Work out the finished part from the listing and answer in its coordinate system (mm). A direction names the side the tool comes from. Round coordinates to 2 decimals unless told otherwise and drop trailing zeros. Write each loop counter-clockwise with the first axis right and the second up, starting at its lowest first coordinate (ties: lowest second). Pieces come first, ordered by that corner, then holes. Notation, with made-up numbers: (24, 7.25) - (56, 7.25) arc R6 cw to (56, 14.25) - close; hole circle Ø11 at (-39.75, 17). An arc over 180 degrees is marked (long way). Write item = value, one per line. Start each with the question number.
Autodesk Inventor part; units mm, degrees
ref_plane "Arbeitsebene1" through (50, 151.9868, 0) normal (-1, 0, 0) x (0, 0, 1)
ref_plane "YZ Plane" through (0, 0, 0) normal (1, 0, 0) x (0, 1, 0)
ref_plane "XZ Plane" through (0, 0, 0) normal (0, 1, 0) x (-1, 0, 0)
sketch "Skizze1" plane through (0, 0, 0) normal (0, 0, 1) x (1, 0, 0)
  line L0 (-33.0017, 0) -> (83.0017, 0) construction
  circle A0 centre (50, 151.9868) radius 16
  line L1 (66, 151.9868) -> (66, 221.9868)
  line L2 (34, 151.9868) -> (34, 221.9868)
  line L3 (50, 151.9868) -> (50, 237.9868) construction
  line L4 (50, 151.9868) -> (50, 167.9868) construction
  line L5 (34, 151.9868) -> (66, 151.9868) construction
  line L6 (-16, 0) -> (-16, 50)
  line L7 (16, 0) -> (16, 50)
  line L8 (-16, 50) -> (16, 50) construction
  circle A1 centre (0, 50) radius 16 construction
  line L9 (-14.2566, 57.2629) -> (34, 151.9868)
  arc A2 (-14.2566, 57.2629) -> (-16, 50) centre (0, 50) ccw
  line L10 (16, 50) -> (64.2566, 144.7239)
  arc A3 (64.2566, 144.7239) -> (66, 151.9868) centre (50, 151.9868) ccw
  line L11 (0, 50) -> (50, 151.9868) construction
  circle A4 centre (50, 221.9868) radius 16
  circle A5 centre (50, 221.9868) radius 9.5
  circle A6 centre (50, 151.9868) radius 9.5
  line L12 (0, 0) -> (0, 5) construction
  circle A7 centre (50, 151.9868) radius 12.75 construction
  circle A8 centre (50, 221.9868) radius 12.75 construction
  line L13 (0, 0) -> (50, 221.9868) construction
  circle A9 centre (50, 221.9868) radius 10.5
  circle A10 centre (50, 151.9868) radius 10.5
  circle A11 centre (50, 151.9868) radius 12
  circle A12 centre (50, 221.9868) radius 12
  line L14 (-16, 0) -> (-16, -17)
  line L15 (-16, -17) -> (16, -17)
  line L16 (16, -17) -> (16, 0)
  circle A13 centre (0, 0) radius 5
  line L17 (-1.5, -4.7697) -> (-1.5, -17)
  line L18 (1.5, -17) -> (1.5, -4.7697)
  line L19 (-16, 0) -> (16, 0) construction
  arc A14 (16, 0) -> (-16, 0) centre (0, 0) ccw
  line L20 (-1.5, 4.7697) -> (-1.5, 10.7697)
  arc A15 (1.5, 10.7697) -> (-1.5, 10.7697) centre (0, 10.7697) ccw
  line L21 (1.5, 10.7697) -> (1.5, 4.7697)
  line L22 (1.5, 4.7697) -> (-1.5, 4.7697)
  line L23 (0, 12.2697) -> (0, 40)
  line L24 (0, 40) -> (16, 40)
  line L25 (0, 33) -> (-4.8, 35)
  line L26 (-4.8, 35) -> (-4.8, 21)
  line L27 (-4.8, 21) -> (0, 23)
  line L28 (-4.8, 28) -> (0, 28) construction
  line L29 (-4.8, 30.5) -> (0, 30.5) construction
  line L30 (-4.8, 25.5) -> (0, 25.5) construction
  circle A16 centre (-10.5, 0) radius 1.55
  circle A17 centre (10.5, 0) radius 1.55
  line L31 (0, 0) -> (50, 151.9868) construction
  point P0 (26.4122, 103.8739)
  point P1 (50, 186.9868)
  point P2 (50, 164.7368)
  point P3 (38.9582, 145.6118)
  point P4 (61.0418, 145.6118)
  point P5 (50, 234.7368)
  point P6 (38.9582, 215.6118)
  point P7 (61.0418, 215.6118)
  point P8 (-5, 0)
  dimension "d69" = 25.5
  dimension "ParallelHebel_Passflansch_HoleDia" = 25.5
  dimension "d36" = 0
  dimension "ParallelHebel_Gabelgelenk_OuterDia" = 32
  dimension "VerticalDistance" = 70
  dimension "d42" = 60
  dimension "d43" = 19
  dimension "Nadellager_OuterDia" = 19
  dimension "d45" = 35
  dimension "d67" = 360
  dimension "d72" = 360
  dimension "Distanze_daVinciHead_Pivot" = 221.9868
  dimension "d88" = 21
  dimension "d91" = 24
  dimension "d92" = 24
  dimension "d97" = 151.9868
  dimension "Support_Link_Length" = 160
  dimension "d100" = 10
  dimension "d101" = 3
  dimension "d102" = 0
  dimension "d103" = 17
  dimension "d105" = 32
  dimension "d125" = 50
  dimension "d128" = 50
  dimension "d138" = 6
  dimension "d139" = 10
  dimension "d142" = 14
  dimension "d143" = 10
  dimension "d144" = 2.5
  dimension "d145" = 5
  dimension "d146" = 4.8
  dimension "d147" = 28
  dimension "d173" = 11
  dimension "d174" = 5.5
  dimension "d175" = 3.1
  dimension "d178" = 71.79
extrude "Extrusion2" add sketch "Skizze1" along normal blind 8 contours A0 | A0 L2 A4 L1 | A0 L10 L7 L24 L23 L25 L26 L27 A14 L6 A2 L9 | A4 | L7 A14 L23 L24 | A14 L23 A15 L20 A13 L17 L15 L14 | L16 L15 L18 A13 L21 A15 L23 A14 | L23 L27 L26 L25 | A15 L21 A13 L20 | A9 | A10 | A11 | A12 | A16 | A17
fillet "Rundung1" radius 25 2 edges at (34, 151.9868, 4) (16, 50, 4)
hole "Bohrung2" at (50, 186.9868, 0) at (26.4122, 103.8739, 0) direction (0, 0, 1) diameter 8 end through all
ref_plane "Arbeitsebene1" through (50, 151.9868, 0) normal (-1, 0, 0) x (0, 0, 1)
extrude "Extrusion6" cut sketch "Skizze1" along normal blind 1 contours A5 | A9 | A10 | A11 | A12
extrude "Extrusion7" cut sketch "Skizze1" along normal blind 1 from surface at 1 contours A9 | A10
sketch "Skizze8" plane through (0, 0, 8) normal (0, 0, 1) x (1, 0, 0)
  circle A0 centre (50, 186.9868) radius 4
  circle A1 centre (26.4122, 103.8739) radius 4
  arc A2 (64.2566, 144.7239) -> (66, 151.9868) centre (50, 151.9868) ccw
  line L0 (66, 151.9868) -> (66, 221.9868)
  arc A3 (66, 221.9868) -> (34, 221.9868) centre (50, 221.9868) ccw
  line L1 (34, 221.9868) -> (34, 157.988)
  arc A4 (31.2759, 146.6396) -> (34, 157.988) centre (9, 157.988) ccw
  line L2 (31.2759, 146.6396) -> (-14.2566, 57.2629)
  arc A5 (-14.2566, 57.2629) -> (-16, 50) centre (0, 50) ccw
  line L3 (-16, 50) -> (-16, -17)
  line L4 (-16, -17) -> (-1.5, -17)
  line L5 (-1.5, -17) -> (-1.5, -4.7697)
  arc A6 (1.5, -4.7697) -> (-1.5, -4.7697) centre (0, 0) ccw
  line L6 (1.5, -4.7697) -> (1.5, -17)
  line L7 (1.5, -17) -> (16, -17)
  line L8 (16, -17) -> (16, 43.9989)
  arc A7 (18.7241, 55.3472) -> (16, 43.9989) centre (41, 43.9989) ccw
  line L9 (18.7241, 55.3472) -> (64.2566, 144.7239)
  circle A8 centre (50, 151.9868) radius 9.5
  circle A9 centre (50, 221.9868) radius 9.5
extrude "Extrusion9" add sketch "Skizze8" along normal blind 5
sketch "Skizze5" plane through (-1.5, -17, 0) normal (1, 0, 0) x (0, 0, -1)
  line L0 (0, 0) -> (0, 12.2303) construction
  line L1 (0, 12.2303) -> (-13, 12.2303) construction
  line L2 (0, 0) -> (-13, 0) construction
  line L3 (-13, 12.2303) -> (0, 0) construction
  line L4 (-13, 0) -> (0, 12.2303) construction
  line L5 (-13, 0) -> (-13, 12.2303) construction
  point P0 (0, 17)
  point P1 (-6.5, 6.1152)
extrude "Extrusion11" add sketch "Skizze1" along normal up to surface (13 mm away) separate body contours L7 A14 L23 L24 | L16 L15 L18 A13 L21 A15 L23 A14 | L23 L27 L26 L25 | A17
extrude "Extrusion10" cut sketch "Skizze1" along normal up to surface (13 mm away) contours L7 A14 L23 L24 | L16 L15 L18 A13 L21 A15 L23 A14 | L23 L27 L26 L25 | A15 L21 A13 L20 | A17 bodies 1
hole "Bohrung4" at (-1.5, -10.8848, 6.5) direction (-1, 0, 0) diameter 3.242 end through all bodies 1
sketch "Skizze9" plane through (16, -17, 0) normal (1, 0, 0) x (0, 0, -1)
  point P0 (0, 17)
  point P1 (-6.5, 6.1152)
hole "Bohrung6" at (16, -10.8848, 6.5) direction (-1, 0, 0) diameter 4.5 depth 17.5 counterbore diameter 8 counterbore depth 4.5 bodies 2
ref_plane "Arbeitsebene2" through (-4.8, 72.7467, 13) normal (-1, 0, 0) x (0, 1, 0)
sketch "Skizze12" plane through (-4.8, 72.7467, 13) normal (-1, 0, 0) x (0, 1, 0)
  line L0 (-44.7467, 13) -> (-44.7467, 6.5) construction
  line L1 (-22.7467, 13) -> (-89.7467, 13) construction
  line L2 (-22.7467, 0) -> (-89.7467, 0) construction
  point P0 (-72.7467, 13)
  point P1 (-44.7467, 13)
  dimension "d150" = 13
  dimension "d151" = 6.5
sketch "Skizze13" plane through (16, -17, 0) normal (1, 0, 0) x (0, 0, -1)
  point P0 (0, 17)
  point P1 (-6.5, 45)
hole "Bohrung7" at (-4.8, 28, 6.5) direction (-1, 0, 0) diameter 3.242 end through all bodies 1
hole "Bohrung8" at (16, 28, 6.5) direction (-1, 0, 0) diameter 4.5 end through all counterbore diameter 8 counterbore depth 4.5 bodies 2
extrude "Extrusion12" cut sketch "Skizze1" along normal through all contours A17 bodies 2
delete faces "Fläche löschen1" heal no whole lump yes faces at (-8.5333, 28.26, 4.9)
thicken "Thicken1" operation add thickness 0.15 both sides no extend neighbours yes toward (-0.3846154, -0.9230769, 0) bodies 2 faces at (-1.6, 33.6667, 4.3333) (-4.8, 22.5888, 6.5904) (-3.2, 21.6667, 4.3333) (0, 19.4232, 8.6667) (0, 37.6667, 4.3333)
equation "\"NKX_10_RiadialPart_Dia\" = 19"
equation "\"Lager_Bohrung_Durchmesser\" = 19"
equation "\"Lager_Einbautiefe\" = 5"
properties part number "ParallelSystem_ProximalPart_Driven_Counterpart" material "PBT-Kunststoff"
1. Consider line 1 (Y direction, x = 13.85, z = 6.5); line 2 (Y direction, x = 8.25, z = 6.5); line 3 (X direction, y = 0, z = 4.25). Determine where each line is inside the solid, lowest interval first.
2. Find section B-B on x = 10.5. Give the vertices of the cut face in (y, z).
3. For a pull along Z with two mould halves and no side action, classify faces 1 (the face through (11.5, -9, 5)), 2 (the face through (-4.65, 28, 4)), 3 (the face through (8, 12, 13)) as released by +Z, released by -Z, zero draft, split by the parting line, or undercut.
4. Find section A-A on z = 6.5. Give the number of separate pieces and of enclosed holes in the cut face, plus the area to 3 significant figures.
5. Each of these flat-tipped pins is pushed along its axis until it touches: pin 1 (5 mm diameter, centred on y = 28, z = 6.5, fed in from -X); pin 2 (2.5 mm diameter, centred on y = 29, z = 5.5, fed in from +X); pin 3 (5 mm diameter, centred on y = 15, z = 8.5, fed in from -X); pin 4 (2.5 mm diameter, centred on y = -10.88, z = 6.5, fed in from +X). Where does it stop, or does it pass through?
6. Which of the six approach directions +Z, -Z, +X, -X, +Y, -Y give full straight-line access (tool end or side, diameter ignored) to faces 4 (the face through (13.72, -6.98, 7.37)), 5 (the face through (0.15, 18, 6)), 6 (the face through (-2.216, 33.761, 6.409)), 7 (the face through (1.5, 8, 6))?
7. Find section C-C on z = 1.5. Give the vertices of the cut face in (x, y) (3 decimals).
8. Find section D-D on y = 0. Give the vertices of the cut face in (x, z), plus the area to 3 significant figures.
Answer key:
q1.line_1 = -17 to -14.88, -6.88 to 24, 32 to 40
q1.line_2 = -17 to -13.13, -8.63 to 25.75, 30.25 to 40
q1.line_3 = 5 to 8.95, 12.05 to 16
q2.outline = (-17, 0) - (-1.55, 0) - (-1.55, 13) - (-17, 13) - close; (1.55, 0) - (40, 0) - (40, 13) - (1.55, 13) - close; hole circle Ø4.5 at (-10.88, 6.5); hole circle Ø4.5 at (28, 6.5)
q3.face_1 = undercut
q3.face_2 = zero draft
q3.face_3 = released by +Z
q4.separate_pieces = 3
q4.enclosed_holes = 1
q4.area = 698 mm²
q5.pin_1 = -4.65
q5.pin_2 = 11.5
q5.pin_3 = 0.15
q5.pin_4 = through
q6.face_4 = +X
q6.face_5 = +Z, -Z, -Y
q6.face_6 = +Z, -Z, +Y
q6.face_7 = +Z, -Z, -X, -Y
q7.outline = (-4.65, 21.225) - (0.15, 23.225) - (0.15, 12.262) arc R1.5 cw to (1.5, 10.77) - (1.5, 4.77) arc R5 cw to (1.5, -4.77) - (1.5, -17) - (16, -17) - (16, 40) - (0.15, 40) - (0.15, 32.775) - (-4.65, 34.775) - close; hole circle Ø3.1 at (10.5, 0)
q8.outline = (5, 0) - (8.95, 0) - (8.95, 13) - (5, 13) - close; (12.05, 0) - (16, 0) - (16, 13) - (12.05, 13) - close
q8.area = 103 mm²
